The model under review builds one solid part; all positions refer to its coordinate system, in mm. Face numbers are marked on the shaded views. A direction names the side the tool comes from. Coordinates: 2 decimals unless noted, no trailing zeros. Loops run counter-clockwise (first coordinate to the right, second up) from the corner with the lowest first, then second, coordinate; pieces in that order, holes last. Notation, with made-up numbers: M 87.25,77.5 L 114.25,77.5 A12 cw 114.25,95.5 Z; hole C 23,21.5 d8. An arc over 180 degrees is marked long. Use one line per item in the form item = value.
```python
from build123d import *

# Parameters (mm, degrees)
SKETCH1_W           = 55
SKETCH1_H           = 35
BOSS_EXTRUDE1_DEPTH = 3
SKETCH2_W           = 55
SKETCH2_H           = 82
BOSS_EXTRUDE2_DEPTH = 3
BOSS_EXTRUDE3_DEPTH = 3
BOSS_EXTRUDE4_DEPTH = 3
SKETCH5_R           = 13
SKETCH5_R_2         = 2.15
CUT_EXTRUDE1_DEPTH  = 3


with BuildPart() as part:
    # Sketch1 → Boss-Extrude1 (new body)
    with BuildSketch(Plane(origin=(0, 0, 0), x_dir=(1, 0, 0), z_dir=(0, 1, 0))):
        Rectangle(SKETCH1_W, SKETCH1_H)
    extrude(amount=BOSS_EXTRUDE1_DEPTH)

    # Sketch2 → Boss-Extrude2 (add)
    with BuildSketch(Plane.XY.offset(17.5)):
        with Locations((0, -14)):
            Rectangle(SKETCH2_W, SKETCH2_H)
    extrude(amount=BOSS_EXTRUDE2_DEPTH)

    # Sketch3 → Boss-Extrude3 (add)
    with BuildSketch(Plane(origin=(27.5, 0, 0), x_dir=(0, 0, -1), z_dir=(1, 0, 0))):
        Polygon((-17.5, 0), (12.5, 0), (-17.5, -50), align=None)
    extrude(amount=-BOSS_EXTRUDE3_DEPTH)

    # Sketch4 → Boss-Extrude4 (add)
    with BuildSketch(Plane.ZY.offset(27.5)):
        Polygon((-12.5, 0), (17.5, 0), (17.5, -50), align=None)
    extrude(amount=-BOSS_EXTRUDE4_DEPTH)

    # Sketch5 → Cut-Extrude1 (cut)
    with BuildSketch(Plane(origin=(0, 0, 17.5), x_dir=(-1, 0, 0), z_dir=(0, 0, -1))):
        with Locations((0, -25)):
            Circle(SKETCH5_R)
        with Locations((12.374368671, -12.625631329)):
            Circle(SKETCH5_R_2)
        with Locations((12.374368671, -37.374368671)):
            Circle(SKETCH5_R_2)
        with Locations((-12.374368671, -37.374368671)):
            Circle(SKETCH5_R_2)
        with Locations((-12.374368671, -12.625631329)):
            Circle(SKETCH5_R_2)
    extrude(amount=-CUT_EXTRUDE1_DEPTH, mode=Mode.SUBTRACT)


solid = part.part
```
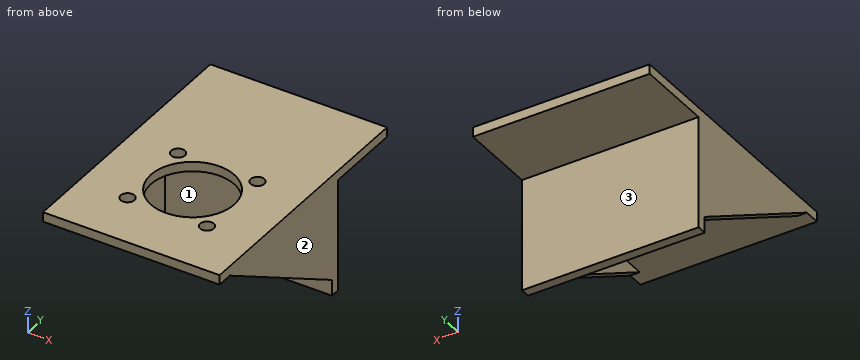
1. Add section A-A (y = -25). State the section outline as (x, z) points.
Response values:
outline = M -27.5,2.5 L -24.5,2.5 L -24.5,17.5 L -13,17.5 L -13,20.5 L -27.5,20.5 Z; M 13,17.5 L 24.5,17.5 L 24.5,2.5 L 27.5,2.5 L 27.5,20.5 L 13,20.5 Z
2. Add section C-C (z = -5). State the section outline as (x, y) points.
Response values:
outline = M -27.5,-12.5 L -24.5,-12.5 L -24.5,0 L 24.5,0 L 24.5,-12.5 L 27.5,-12.5 L 27.5,3 L -27.5,3 Z
3. Add section B-B (x = 5). State the section outline as (y, z) points.
Response values:
outline = M -55,17.5 L -37,17.5 L -37,20.5 L -55,20.5 Z; M -13,17.5 L 0,17.5 L 0,-17.5 L 3,-17.5 L 3,17.5 L 27,17.5 L 27,20.5 L -13,20.5 Z
4. Wall thickness on line 1 along X through (y, z) = (-48, 17); line 2 along Y through (x, z) = (0, 18.15); line 3 along Y through (x, z) = (14, -5): over which ranges is each line inside the solid? List them lowest first. Write a range as from..to.
Response values:
line_1 = -27.5..-24.5, 24.5..27.5
line_2 = -55..-38, -12..27
line_3 = 0..3
5. Add section D-D (y = -43). State the section outline as (x, z) points, then the cut area to 3 significant figures.
Response values:
outline = M -27.5,13.3 L -24.5,13.3 L -24.5,17.5 L 24.5,17.5 L 24.5,13.3 L 27.5,13.3 L 27.5,20.5 L -27.5,20.5 Z
area = 190 mm^2
6. Machinability: for the marked faces 1, 2 and 3, which of the approach directions +Z, -Z, +X, -X, +Y, -Y give a long, thin tool a straight path to every point of the face, cutting with its end or side? Answer none if there is none.
Response values:
face_1 = -Z, -Y
face_2 = +Z, -Z, +X, +Y, -Y
face_3 = -Z, +X, -X, +Y
7. Insertion check: P1, Ø4, axis at y = -25.5, z = 1.5, coming from the +X side; P2, Ø17.5, axis at x = 3.5, z = -6.5, coming from the -Y side; P3, Ø10.5, axis at x = 9, z = 5, coming from the +Y side; P4, Ø12, axis at x = 10, y = 13.5, coming from the -Z side. Each pin has a flat end and moves straight along its axis. Give the tip position at first contact, or say it passes through.
Response values:
P1 = 27.5
P2 = 0
P3 = 3
P4 = 17.5
